Autodesk Inventor part; units mm, degrees
ref_plane "Work Plane1" through (5.75, 0, 0) normal (1, 0, 0) x (0, 1, 0)
ref_plane "XZ Plane" through (0, 0, 0) normal (0, 1, 0) x (-1, 0, 0)
ref_plane "XY Plane" through (0, 0, 0) normal (0, 0, 1) x (1, 0, 0)
sketch "Sketch1" plane through (0, 0, 0) normal (1, 0, 0) x (0, 1, 0)
  circle A0 centre (0, 0) radius 3
  dimension "d0" = 6
extrude "Extrusion1" add sketch "Sketch1" along normal blind 11.5
sketch "Sketch2" plane through (11.5, 0, 0) normal (1, 0, 0) x (0, 0, -1)
  circle A0 centre (0, 0) radius 1.5
  dimension "d3" = 3
extrude "Extrusion2" add sketch "Sketch2" along normal blind 3
sketch "Sketch3" plane through (0, 0, 0) normal (0, 1, 0) x (-1, 0, 0)
  line L0 (-14.5, 1.5) -> (-14.5, -1.5)
  line L1 (-14.5, 0) -> (-14.5, 2)
  line L2 (-14.5, 0) -> (-14.5, -2)
  line L3 (-14.5, -2) -> (-16, -2)
  line L4 (-14.5, 2) -> (-16, 2)
  line L5 (-16, 2) -> (-16, -2)
  point P0 (0, 0)
  dimension "d6" = 2
  dimension "d7" = 2
  dimension "d8" = 1.5
extrude "Extrusion3" add sketch "Sketch3" along normal mid plane 4
fillet "Fillet1" radius 2 4 edges at (15.25, 2, -2) (15.25, 2, 2) (15.25, -2, 2) (15.25, -2, -2)
fillet "Fillet2" radius 2 3 edges at (16, 0, -2) (16, 1.4142, -1.4142) (16, 2, 0)
ref_plane "Work Plane1" through (5.75, 0, 0) normal (1, 0, 0) x (0, 1, 0)
mirror "Mirror1" about plane through (5.75, 0, 0) normal (1, 0, 0) of "Extrusion2"
sketch "Sketch4" plane through (0, 0, 0) normal (0, 1, 0) x (-1, 0, 0)
  line L0 (3, 1.5) -> (3, -1.5)
  line L1 (3, 0) -> (3, 2)
  line L2 (3, 2) -> (3, -2)
  line L3 (3, -2) -> (4.5, -2)
  line L4 (4.5, -2) -> (4.5, 2)
  line L5 (4.5, 2) -> (3, 2)
  point P0 (0, 0)
  dimension "d14" = 2
  dimension "d15" = 4
  dimension "d16" = 1.5
extrude "Extrusion4" add sketch "Sketch4" along normal mid plane 4
fillet "Fillet3" radius 2 4 edges at (-3.75, 2, 2) (-3.75, 2, -2) (-3.75, -2, 2) (-3.75, -2, -2)
fillet "Fillet4" radius 2 3 edges at (-4.5, 0, 2) (-4.5, 2, 0) (-4.5, 1.4142, 1.4142)
properties part number "Reverse Gear LInk Rod" material "Copper"
Geometry check sheet. Reference: the model listing, model coordinates, mm. Give positions to 0.01 mm unless a question says otherwise; leave off trailing zeros. Loops run counter-clockwise (first coordinate to the right, second up) from the corner with the lowest first, then second, coordinate; pieces in that order, holes last. Notation, with made-up numbers: (-18, 62) - (8, 62) arc R18 cw to (8, 85) - close; hole circle Ø11 at (7, 49). An arc over 180 degrees is marked (long way). Use CSV: the item, a comma, the result in double quotes. Start each with the question number.
Q1. Release check for a two-part mould opening along X. For faces 1 (the face through (6, -3, 0)), 2 (the face through (0, 1.3, -1.3)) record: +X half, -X half, draft (parallel to the pull), parting line (faces both ways), or undercut.
Q2. Section check A-A, the plane x = 4.25. Record the cut outline in (y, z), and give its area (3 significant figures).
Q3. Section check D-D, the plane x = 12. Record the cut outline in (y, z), and give its area (3 significant figures).
Q4. Section check B-B, the plane y = 1.8. Count the separate pieces of the cut face and the enclosed holes in it, and give its area (3 significant figures).
Q5. Scan lines: probe 1 along X at (y, z) = (0.5, -1.55); probe 2 along X at (y, z) = (-0.4, 1.55); probe 3 along X at (y, z) = (1.25, 2.5). Record each from-to range of solid material in increasing order. Write a range as from..to.
Q6. Go/stop test with flat-tipped pins: pin 1 Ø1.8 at (y, z) = (-1, 0.5) entering from -X; pin 2 Ø2 at (x, z) = (0, -2.5) entering from -Y; pin 3 Ø1.2 at (y, z) = (0.5, 1) entering from +X. Record where each tip stops, or that it passes through.
Findings below:
1,face 1,"draft"
1,face 2,"undercut"
2,outline,"circle Ø6 at (0, 0)"
2,area,"28.3 mm^2"
3,outline,"circle Ø3 at (0, 0)"
3,area,"7.07 mm^2"
4,separate pieces,"3"
4,enclosed holes,"0"
4,area,"56.4 mm^2"
5,probe 1,"x = -3.75..-3, 0..11.5, 14.5..15.25"
5,probe 2,"x = -3.78..-3, 0..11.5, 14.5..15.28"
5,probe 3,"x = 0..11.5"
6,pin 1,"stops at x = -4.49"
6,pin 2,"stops at y = -2.6"
6,pin 3,"stops at x = 15.95"
